Part model, mm, in its own coordinate system. A direction names the side the tool comes from. Round coordinates to 2 decimals unless told otherwise and drop trailing zeros. Order: outer loops, then holes, each group sorted by start corner. A loop starts at its lowest first (then second) coordinate and runs counter-clockwise, first axis right, second up. Notation, with made-up numbers: M 48,-33 L 79,-33 A18 cw 79,-7 Z; hole C -3.5,81 d8. An arc over 180 degrees is marked long. One line per question, with ' | ' between items.
Autodesk Inventor part; units mm, degrees
ref_plane "YZ Plane" through (0, 0, 0) normal (1, 0, 0) x (0, 1, 0)
ref_plane "XZ Plane" through (0, 0, 0) normal (0, 1, 0) x (-1, 0, 0)
ref_plane "XY Plane" through (0, 0, 0) normal (0, 0, 1) x (1, 0, 0)
sketch "Sketch1" plane through (0, 0, 0) normal (0, 0, 1) x (1, 0, 0)
  line L0 (-12.1708, 16.0073) -> (13.2292, 16.0073)
  line L1 (13.2292, 16.0073) -> (13.2292, -34.7927)
  line L2 (13.2292, -34.7927) -> (-12.1708, -34.7927)
  line L3 (-12.1708, -34.7927) -> (-12.1708, 16.0073)
  line L4 (11.9592, 14.7373) -> (-10.9008, 14.7373)
  line L5 (-10.9008, 14.7373) -> (-10.9008, -33.5227)
  line L6 (-10.9008, -33.5227) -> (11.9592, -33.5227)
  line L7 (11.9592, -33.5227) -> (11.9592, 14.7373)
  point P0 (0, 0)
  dimension "d0" = 25.4
  dimension "d1" = 50.8
  dimension "d2" = 1.27
extrude "Extrusion1" add sketch "Sketch1" along normal blind 558.8
sketch "Sketch2" plane through (-12.1708, 16.0073, 0) normal (0, 1, 0) x (1, 0, 0)
  circle A0 centre (12.7, -12.7) radius 1.7272
  line L0 (25.4, 0) -> (0, 0)
  line L1 (0, 0) -> (0, -558.8)
  point P0 (12.1708, 0)
  dimension "d5" = 3.4544
  dimension "d6" = 12.7
  dimension "d7" = 12.7
extrude "Extrusion2" cut sketch "Sketch2" against normal through all
pattern_linear "Rectangular Pattern1" count 56 spacing 25.4 along (0, 0, 1) of "Extrusion2"
equation "\"d3\" = d13"
equation "\"d10\" = d14"
equation "\"d13\" = 558.8"
equation "\"d14\" = d13"
properties part number "VersaFrame( perimiter peices A)"
1) Which spindle directions (+Z, -Z, +X, -X, +Y, -Y) get a long thin tool onto all of the face, cutting with end or side? Do faces 1 (the face through (-12, -9, 0)), 2 (the face through (11.959, -10, 275)). Say none if no direction does.
The answers:
face 1: -Z, +X, -X, +Y, -Y | face 2: +Z, -Z
2) Drop a flat-ended pin along its axis: pin 1 (5.5 mm diameter, centred on x = 0.53, z = 215.9, fed in from +Y). Give the stop position or say it passes through.
The answers:
pin 1: stops at y = 16.01
3) Two-plate mould, pull along X, no slides. Class faces 3 (the face through (1, -34.793, 275)), 4 (the face through (-10.901, -9, 275)), 5 (the face through (13.229, -9, 275)): released by +X, released by -X, zero draft, split by the parting line, or undercut.
The answers:
face 3: zero draft | face 4: undercut | face 5: released by +X
4) Probe line 1 (X direction, y = 15.45, z = 63.5); line 2 (X direction, y = -24.5, z = 476); line 3 (Y direction, x = -5.75, z = 519). List the from-to ranges inside material, lowest first. Write a range as [from, to].
The answers:
line 1: x = [-12.17, -1.2], [2.26, 13.23] | line 2: x = [-12.17, -10.9], [11.96, 13.23] | line 3: y = [-34.79, -33.52], [14.74, 16.01]
5) Saw through at A-A (y = 7). List the corners of the cut face in (x, z), plus the area to 3 significant figures.
The answers:
outline: M -12.17,0 L -10.9,0 L -10.9,558.8 L -12.17,558.8 Z; M 11.96,0 L 13.23,0 L 13.23,558.8 L 11.96,558.8 Z | area: 1,420 mm²
6) Saw through at B-B (z = 305). List the corners of the cut face in (x, y).
The answers:
outline: M -12.17,-34.79 L 13.23,-34.79 L 13.23,16.01 L -12.17,16.01 Z; hole M -10.9,-33.52 L 11.96,-33.52 L 11.96,14.74 L -10.9,14.74 Z
